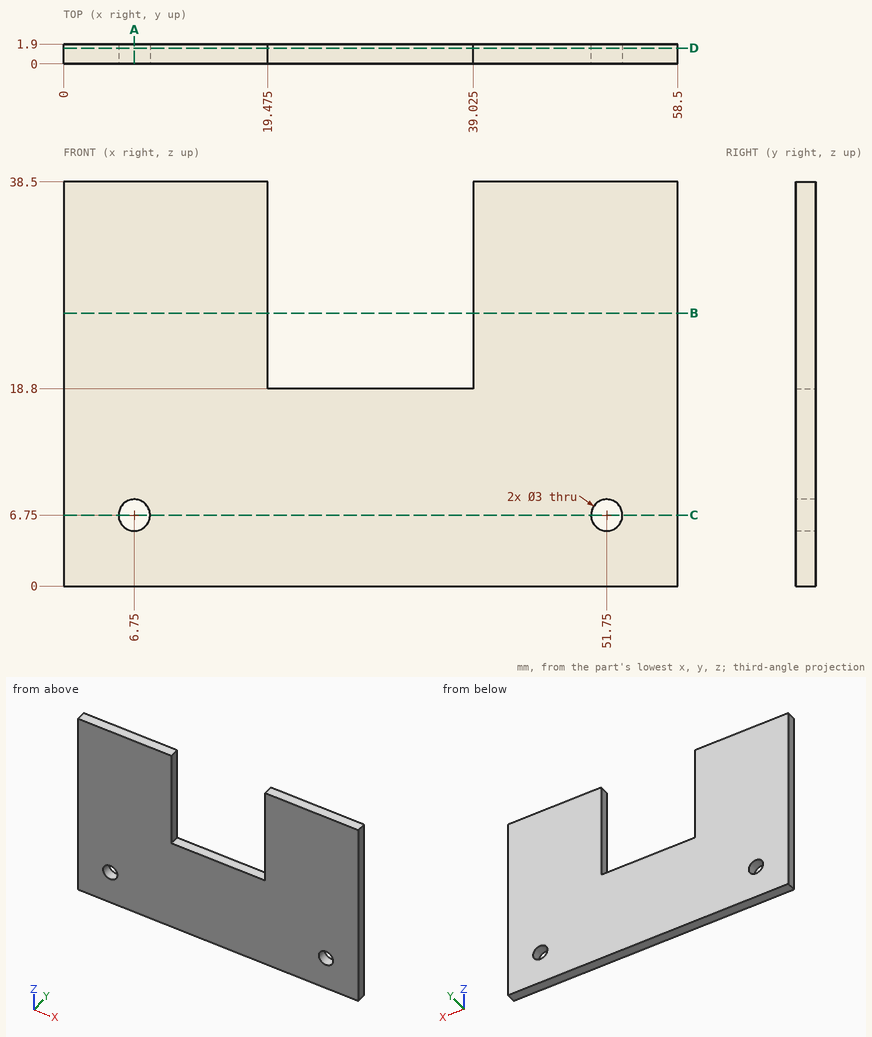
The figure shows three views and two pictorial views of one solid part (mm, origin at its lowest corner). Answer the questions. Round coordinates to 2 decimals unless told otherwise and drop trailing zeros. Order: outer loops, then holes, each group sorted by start corner. A loop starts at its lowest first (then second) coordinate and runs counter-clockwise, first axis right, second up. Notation, with made-up numbers: (27.5, -16) -> (54.5, -16) arc R25 ccw to (54.5, 3) -> close; hole circle Ø6 at (7, 48.5). An arc over 180 degrees is marked (long way). Put each result on its own line as item: value.
Q1. Section B-B, the plane z = 26 is taken. Write down the section's boundary in (x, y) (3 decimals), and give its area (3 significant figures).
Results list:
outline: (0, 0) -> (19.475, 0) -> (19.475, 1.9) -> (0, 1.9) -> close; (39.025, 0) -> (58.5, 0) -> (58.5, 1.9) -> (39.025, 1.9) -> close
area: 74.0 mm^2
Q2. Consider line 1 along X through (y, z) = (0.7, 32.5) (3 decimals); line 2 along X through (y, z) = (0.55, 6.75); line 3 along Z through (x, y) = (51, 0.85). Determine where each line is inside the solid, lowest interval first.
Results list:
line 1: 0 to 19.475, 39.025 to 58.5
line 2: 0 to 5.25, 8.25 to 50.25, 53.25 to 58.5
line 3: 0 to 5.45, 8.05 to 38.5
Q3. Each of these flat-tipped pins is pushed along its axis until it touches: P1, Ø1, axis at x = 42.5, z = 22, coming from the -Y side; P2, Ø0.6, axis at x = 34, y = 1.5, coming from the +Z side; P3, Ø2.5, axis at x = 6.75, z = 6.75, coming from the +Y side. Where does it stop, or does it pass through?
Results list:
P1: y = 0
P2: z = 18.8
P3: through
Q4. Section A-A, the plane x = 6.75 is taken. Write down the section's boundary in (y, z), and give its area (4 significant figures).
Results list:
outline: (0, 0) -> (1.9, 0) -> (1.9, 5.25) -> (0, 5.25) -> close; (0, 8.25) -> (1.9, 8.25) -> (1.9, 38.5) -> (0, 38.5) -> close
area: 67.45 mm^2
Q5. Section C-C, the plane z = 6.75 is taken. Write down the section's boundary in (x, y), and give its area (4 significant figures).
Results list:
outline: (0, 0) -> (5.25, 0) -> (5.25, 1.9) -> (0, 1.9) -> close; (8.25, 0) -> (50.25, 0) -> (50.25, 1.9) -> (8.25, 1.9) -> close; (53.25, 0) -> (58.5, 0) -> (58.5, 1.9) -> (53.25, 1.9) -> close
area: 99.75 mm^2
Q6. Section D-D, the plane y = 1.5 is taken. Write down the section's boundary in (x, z) (3 decimals).
Results list:
outline: (0, 0) -> (58.5, 0) -> (58.5, 38.5) -> (39.025, 38.5) -> (39.025, 18.8) -> (19.475, 18.8) -> (19.475, 38.5) -> (0, 38.5) -> close; hole circle Ø3 at (6.75, 6.75); hole circle Ø3 at (51.75, 6.75)
